Study the drawing (mm; zero at the part's minimum x, y, z) and answer. A direction names the side the tool comes from. Give positions to 0.01 mm unless a question says otherwise; leave off trailing zeros. Order: outer loops, then holes, each group sorted by start corner. A loop starts at its lowest first (then second) coordinate and runs counter-clockwise, first axis right, second up. Notation, with made-up numbers: (6, 58) - (28, 58) arc R10 cw to (28, 63) - close; hole circle Ø1 at (-36, -16). An arc over 180 degrees is marked (long way). Return JSON: item names as keys, results as strings.
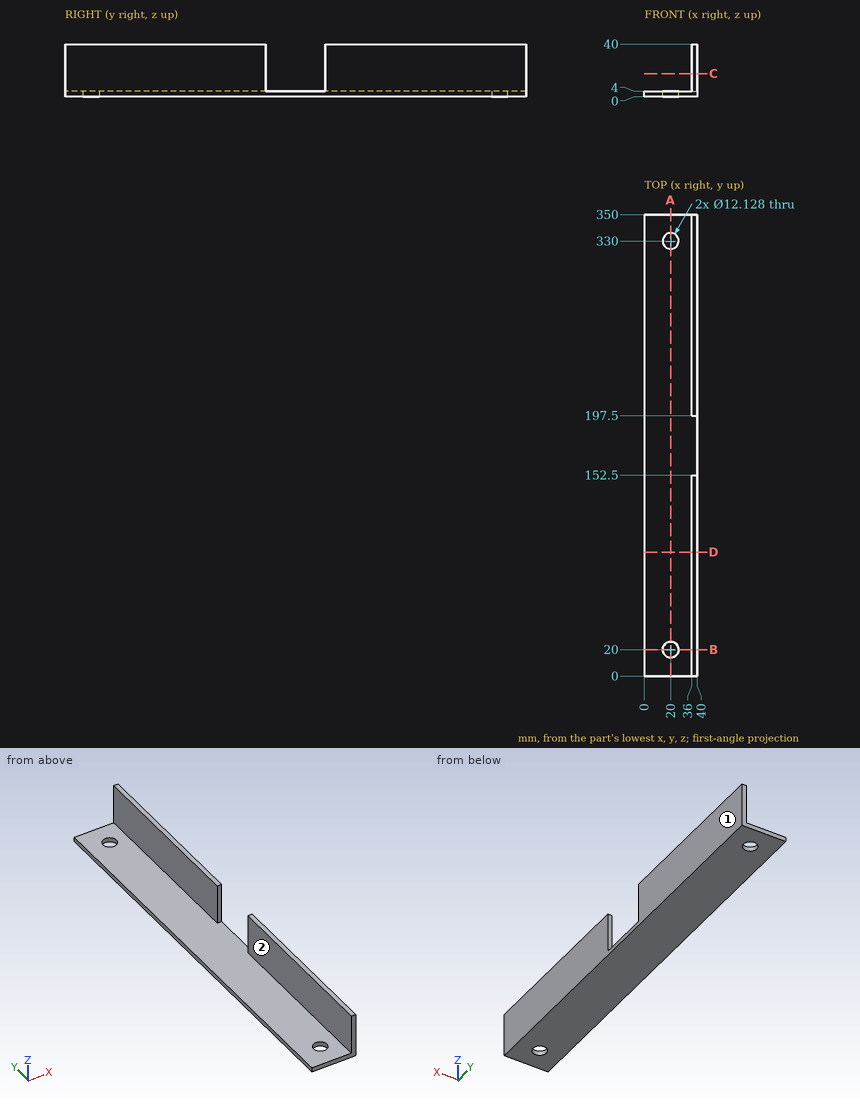
Q1. For the marked faces 1 and 2, determine the directions among +Z, -Z, +X, -X, +Y, -Y from which every point of the face is accessible in a straight line to the end or side of a thin tool.
Values:
{"face 1": "+Z, -Z, +X, +Y, -Y", "face 2": "+Z, -X, +Y, -Y"}
Q2. Consider L1, parallel to X at y = 330, z = 2; L2, parallel to Z at x = 4.5, y = 118; L3, parallel to X at y = 264, z = 27.5. Determine where each line is inside the solid, lowest interval first.
Values:
{"L1": "x = 0 to 13.94, 26.06 to 40", "L2": "z = 0 to 4", "L3": "x = 36 to 40"}
Q3. A cutting plane is placed at D-D (y = 94). Write down the section's boundary in (x, z).
Values:
{"outline": "(0, 0) - (40, 0) - (40, 40) - (36, 40) - (36, 4) - (0, 4) - close"}
Q4. Given pin 1 (6 mm diameter, centred on x = 28, y = 35.5, fed in from -Z); pin 2 (4 mm diameter, centred on x = 9, y = 269.5, fed in from +Z); pin 3 (7.5 mm diameter, centred on x = 20, y = 330, fed in from -Z); pin 4 (1.5 mm diameter, centred on y = 64, z = 12, fed in from -X), each flat-ended and moving along its own axis, determine where each tip first touches the part or whether it passes through.
Values:
{"pin 1": "stops at z = 0", "pin 2": "stops at z = 4", "pin 3": "passes through", "pin 4": "stops at x = 36"}
Q5. A cutting plane is placed at C-C (z = 17.5). Write down the section's boundary in (x, y).
Values:
{"outline": "(36, 0) - (40, 0) - (40, 152.5) - (36, 152.5) - close; (36, 197.5) - (40, 197.5) - (40, 350) - (36, 350) - close"}
Q6. A cutting plane is placed at A-A (x = 20). Write down the section's boundary in (y, z).
Values:
{"outline": "(0, 0) - (13.94, 0) - (13.94, 4) - (0, 4) - close; (26.06, 0) - (323.94, 0) - (323.94, 4) - (26.06, 4) - close; (336.06, 0) - (350, 0) - (350, 4) - (336.06, 4) - close"}
Q7. A cutting plane is placed at B-B (y = 20). Write down the section's boundary in (x, z).
Values:
{"outline": "(0, 0) - (13.94, 0) - (13.94, 4) - (0, 4) - close; (26.06, 0) - (40, 0) - (40, 40) - (36, 40) - (36, 4) - (26.06, 4) - close"}
